```python
from build123d import *

# Parameters (mm, degrees)
SKETCH1_R           = 139.7
SKETCH1_R_2         = 107.95
SKETCH1_R_3         = 3.175
BOSS_EXTRUDE1_DEPTH = 139.7
SKETCH6_R           = 139.7
SKETCH6_R_2         = 3.175
SKETCH6_R_3         = 114.286339031
CUT_EXTRUDE4_DEPTH  = 127


with BuildPart() as part:
    # Sketch1 → Boss-Extrude1 (new body, symmetric)
    with BuildSketch(Plane(origin=(0, 0, 0), x_dir=(1, 0, 0), z_dir=(0, 1, 0))):
        Circle(SKETCH1_R)
        Circle(SKETCH1_R_2, mode=Mode.SUBTRACT)
        with Locations((0, 127)):
            Circle(SKETCH1_R_3, mode=Mode.SUBTRACT)
        with Locations((127, 0)):
            Circle(SKETCH1_R_3, mode=Mode.SUBTRACT)
        with Locations((63.5, 109.985226281)):
            Circle(SKETCH1_R_3, mode=Mode.SUBTRACT)
        with Locations((109.985226281, 63.5)):
            Circle(SKETCH1_R_3, mode=Mode.SUBTRACT)
        with Locations((109.985226281, -63.5)):
            Circle(SKETCH1_R_3, mode=Mode.SUBTRACT)
        with Locations((63.5, -109.985226281)):
            Circle(SKETCH1_R_3, mode=Mode.SUBTRACT)
        with Locations((0, -127)):
            Circle(SKETCH1_R_3, mode=Mode.SUBTRACT)
        with Locations((-63.5, -109.985226281)):
            Circle(SKETCH1_R_3, mode=Mode.SUBTRACT)
        with Locations((-109.985226281, -63.5)):
            Circle(SKETCH1_R_3, mode=Mode.SUBTRACT)
        with Locations((-127, 0)):
            Circle(SKETCH1_R_3, mode=Mode.SUBTRACT)
        with Locations((-109.985226281, 63.5)):
            Circle(SKETCH1_R_3, mode=Mode.SUBTRACT)
        with Locations((-63.5, 109.985226281)):
            Circle(SKETCH1_R_3, mode=Mode.SUBTRACT)
    extrude(amount=BOSS_EXTRUDE1_DEPTH, both=True)

    # Sketch6 → Cut-Extrude4 (cut, symmetric)
    with BuildSketch(Plane(origin=(0, 0, 0), x_dir=(1, 0, 0), z_dir=(0, 1, 0))):
        Circle(SKETCH6_R)
        with Locations((-63.5, 109.985226281)):
            Circle(SKETCH6_R_2, mode=Mode.SUBTRACT)
        with Locations((0, 127)):
            Circle(SKETCH6_R_2, mode=Mode.SUBTRACT)
        with Locations((63.5, 109.985226281)):
            Circle(SKETCH6_R_2, mode=Mode.SUBTRACT)
        with Locations((109.985226281, 63.5)):
            Circle(SKETCH6_R_2, mode=Mode.SUBTRACT)
        with Locations((127, 0)):
            Circle(SKETCH6_R_2, mode=Mode.SUBTRACT)
        with Locations((109.985226281, -63.5)):
            Circle(SKETCH6_R_2, mode=Mode.SUBTRACT)
        with Locations((63.5, -109.985226281)):
            Circle(SKETCH6_R_2, mode=Mode.SUBTRACT)
        with Locations((0, -127)):
            Circle(SKETCH6_R_2, mode=Mode.SUBTRACT)
        with Locations((-63.5, -109.985226281)):
            Circle(SKETCH6_R_2, mode=Mode.SUBTRACT)
        with Locations((-109.985226281, -63.5)):
            Circle(SKETCH6_R_2, mode=Mode.SUBTRACT)
        with Locations((-127, 0)):
            Circle(SKETCH6_R_2, mode=Mode.SUBTRACT)
        with Locations((-109.985226281, 63.5)):
            Circle(SKETCH6_R_2, mode=Mode.SUBTRACT)
        Circle(SKETCH6_R_3, mode=Mode.SUBTRACT)
    extrude(amount=CUT_EXTRUDE4_DEPTH, both=True, mode=Mode.SUBTRACT)


solid = part.part
```
Work out the finished part from the listing and answer in its coordinate system (mm). A direction names the side the tool comes from. Coordinates: 2 decimals unless noted, no trailing zeros. Order: outer loops, then holes, each group sorted by start corner. A loop starts at its lowest first (then second) coordinate and runs counter-clockwise, first axis right, second up. Notation, with made-up numbers: (10, -33) - (25, -33) arc R23 ccw to (25, 3) - close; hole circle Ø10 at (-31.5, -3). An arc over 180 degrees is marked (long way). Answer as a JSON object with one key per item and string values.
1. The mould has two halves that part along Z. Classify faces 1 (the face through (-79.56, -1.96, -72.96)), 2 (the face through (-11, -127, -114)), 3 (the face through (-110.86, 133.44, 85.01)): +Z half, -Z half, draft (parallel to the pull), parting line (faces both ways), or undercut.
Output values:
{"face 1": "undercut", "face 2": "draft", "face 3": "parting line"}
2. Find section B-B on x = -27.5. Determine the outline of the cut face in (y, z), plus the area to 3 significant figures.
Output values:
{"outline": "(-139.7, -136.97) - (-127, -136.97) - (-127, -110.93) - (127, -110.93) - (127, -136.97) - (139.7, -136.97) - (139.7, -104.39) - (-139.7, -104.39) - close; (-139.7, 104.39) - (139.7, 104.39) - (139.7, 136.97) - (127, 136.97) - (127, 110.93) - (-127, 110.93) - (-127, 136.97) - (-139.7, 136.97) - close", "area": "4,980 mm²"}
3. Find section A-A on z = 55.5. Determine the outline of the cut face in (x, y).
Output values:
{"outline": "(-128.2, -139.7) - (-92.59, -139.7) - (-92.59, 139.7) - (-128.2, 139.7) - (-128.2, 127) - (-99.91, 127) - (-99.91, -127) - (-128.2, -127) - close; (92.59, -139.7) - (128.2, -139.7) - (128.2, -127) - (99.91, -127) - (99.91, 127) - (128.2, 127) - (128.2, 139.7) - (92.59, 139.7) - close"}
4. Consider line 1 (X direction, y = -133, z = 0) (3 decimals); line 2 (Y direction, x = -64.5, z = 119); line 3 (X direction, y = 134, z = -63). Determine where each line is inside the solid, lowest interval first.
Output values:
{"line 1": "x = -139.7 to -130.175, -123.825 to -107.95, 107.95 to 123.825, 130.175 to 139.7", "line 2": "y = -139.7 to -127, 127 to 139.7", "line 3": "x = -124.69 to -113.12, -106.85 to -87.66, 87.66 to 106.85, 113.12 to 124.69"}
5. Find section C-C on y = -115. Determine the outline of the cut face in (x, z).
Output values:
{"outline": "circle Ø228.57 at (0, 0); hole circle Ø215.9 at (0, 0)"}
6. Each of these flat-tipped pins is pushed along its axis until it touches: P1, Ø10, axis at x = -88, y = -34, coming from the -Z side; P2, Ø6, axis at y = -69.5, z = 53.5, coming from the -X side; P3, Ø10, axis at x = 109.99, z = 63.5, coming from the -Y side; P4, Ø5, axis at x = 23.5, y = -84, coming from the +Z side. Where does it stop, or does it pass through?
Output values:
{"P1": "stops at z = -78.56", "P2": "stops at x = -102.52", "P3": "stops at y = -139.7", "P4": "stops at z = 112.34"}
7. A tool of negligible diameter and unlimited length cuts with its end or side. For faces 4 (the face through (-11, 127, -114)), 5 (the face through (72, -139.7, 82)), from which of +Z, -Z, +X, -X, +Y, -Y can it reach the whole face along a straight path? Write none if from no direction.
Output values:
{"face 4": "none", "face 5": "+Z, -Z, +X, -X, -Y"}
